```python
from build123d import *

# Parameters (mm, degrees)
SKETCH1_W           = 25.4
SKETCH1_H           = 6.35
SKETCH1_H_2         = 24.788235472
BOSS_EXTRUDE1_DEPTH = 6.35
SKETCH2_W           = 25.4
SKETCH2_H           = 6.35
BOSS_EXTRUDE2_DEPTH = 44.45
SKETCH3_R           = 3.175
CUT_EXTRUDE1_DEPTH  = 38.1
SKETCH6_R           = 5
CUT_EXTRUDE2_DEPTH  = 38.488235472
FILLET1_R           = 6.35


with BuildPart() as part:
    # Sketch1 → Boss-Extrude1 (new body)
    with BuildSketch(Plane.XY):
        with Locations((-12.7, -34.313235472)):
            Rectangle(SKETCH1_W, SKETCH1_H)
        with Locations((-12.7, -18.744117736)):
            Rectangle(SKETCH1_W, SKETCH1_H_2)
        with Locations((-12.7, -3.175)):
            Rectangle(SKETCH1_W, SKETCH1_H)
    extrude(amount=BOSS_EXTRUDE1_DEPTH)

    # Sketch2 → Boss-Extrude2 (add)
    with BuildSketch(Plane.XY.offset(6.35)):
        with Locations((-12.7, -3.175)):
            Rectangle(SKETCH2_W, SKETCH2_H)
        with Locations((-12.7, -34.313235472)):
            Rectangle(SKETCH2_W, SKETCH2_H)
    extrude(amount=BOSS_EXTRUDE2_DEPTH)

    # Sketch3 → Cut-Extrude1 (cut)
    with BuildSketch(Plane.XY.offset(6.35)):
        with Locations((-12.7, -26.058235472)):
            Circle(SKETCH3_R)
        with Locations((-12.7, -11.43)):
            Circle(SKETCH3_R)
    extrude(amount=-CUT_EXTRUDE1_DEPTH, mode=Mode.SUBTRACT)

    # Sketch6 → Cut-Extrude2 (cut, through all)
    with BuildSketch(Plane(origin=(0, 0, 0), x_dir=(1, 0, 0), z_dir=(0, 1, 0))):
        with Locations((-16.933333333, -25.4)):
            Circle(SKETCH6_R)
        with Locations((-8.466666667, -38.1)):
            Circle(SKETCH6_R)
    extrude(amount=-CUT_EXTRUDE2_DEPTH, mode=Mode.SUBTRACT)

    # Fillet1
    fillet1_edges = [part.edges().sort_by_distance(p)[0] for p in [
        (0, -3.175, 50.8),
        (-25.4, -3.175, 50.8),
        (-25.4, -34.313235472, 50.8),
        (0, -34.313235472, 50.8),
    ]]
    fillet(fillet1_edges, radius=FILLET1_R)


solid = part.part
```
For this review, take the finished solid that the model builds, in its own axes (mm). A direction names the side the tool comes from. Give positions to 0.01 mm unless a question says otherwise; leave off trailing zeros. Write each loop counter-clockwise with the first axis right and the second up, starting at its lowest first coordinate (ties: lowest second). Pieces come first, ordered by that corner, then holes. Notation, with made-up numbers: M 38,77 L 97,77 A38 ccw 97,116 Z; hole C 64.25,23 d4. An arc over 180 degrees is marked long. Answer as a JSON object with one key per item and string values. Group by question number.
Item 1: For probe 1 along Y at (x, z) = (-12.7, 1.5) (3 decimals); probe 2 along Y at (x, z) = (-5.5, 29); probe 3 along X at (y, z) = (-3.25, 25.4), list the stretches that pass through material, from the lowest coordinate up. Write a range as [from, to].
Item 2: Tool access review of faces 1 (the cylindrical face through (-23.59, -34.27, 48.89)), 2 (the flat face through (-10, -6.35, 28)): name each direction out of +Z, -Z, +X, -X, +Y, -Y from which nothing blocks a thin tool from reaching the whole face with its end or side.
Item 3: For pin 1 Ø8 at (x, y) = (-21, -22.5) entering from +Z, flat-tipped, find the tip position at first contact; note if it passes through.
Item 4: Draft analysis for pull direction X (two halves, no side actions). For faces 3 (the cylindrical face through (-9.55, -34.27, 42.98)), 4 (the flat face through (-13, -18, 0)), 5 (the flat face through (-25.4, -32, 17)), 6 (the cylindrical face through (-9.55, -3.13, 42.98)), state which applies: +X half, -X half, draft (parallel to the pull), parting line (faces both ways), or undercut.
Item 5: Consider section A-A on z = 38.1. Write out the cut boundary in (x, y), plus the area to 3 significant figures.
Item 6: Consider section B-B on y = -11.43. Write out the cut boundary in (x, z) (3 decimals), plus the area to 3 significant figures.
Item 7: Consider section D-D on x = -12.7. Count the separate pieces of the cut face and the enclosed holes in it, plus the area to 3 significant figures.
Item 8: Consider section C-C on z = 15. Write out the cut boundary in (x, y).
Check result:
{
 "1": {"probe 1": "y = [-37.488, -29.233], [-22.883, -14.605], [-8.255, 0]", "probe 2": "y = [-37.49, -31.14], [-6.35, 0]", "probe 3": "x = [-25.4, -21.93], [-11.93, 0]"},
 "2": {"face 1": "+Z, -X, +Y, -Y", "face 2": "+Z, +X, -X"},
 "3": {"pin 1": "stops at z = 6.35"},
 "4": {"face 3": "undercut", "face 4": "draft", "face 5": "-X half", "face 6": "undercut"},
 "5": {"outline": "M -25.4,-37.49 L -13.47,-37.49 L -13.47,-31.14 L -25.4,-31.14 Z; M -25.4,-6.35 L -13.47,-6.35 L -13.47,0 L -25.4,0 Z; M -3.47,-37.49 L 0,-37.49 L 0,-31.14 L -3.47,-31.14 Z; M -3.47,-6.35 L 0,-6.35 L 0,0 L -3.47,0 Z", "area": "196 mm^2"},
 "6": {"outline": "M -25.4,0 L -15.875,0 L -15.875,6.35 L -25.4,6.35 Z; M -9.525,0 L 0,0 L 0,6.35 L -9.525,6.35 Z", "area": "121 mm^2"},
 "7": {"separate pieces": "7", "enclosed holes": "0", "area": "587 mm^2"},
 "8": {"outline": "M -25.4,-37.49 L 0,-37.49 L 0,-31.14 L -25.4,-31.14 Z; M -25.4,-6.35 L 0,-6.35 L 0,0 L -25.4,0 Z"}
}
